Could you check a few things on this drawing? It's one solid part, dimensions in mm from its lowest x, y, z. A direction names the side the tool comes from. Give positions to 0.01 mm unless a question says otherwise; leave off trailing zeros. Write each loop counter-clockwise with the first axis right and the second up, starting at its lowest first coordinate (ties: lowest second). Pieces come first, ordered by that corner, then holes. Notation, with made-up numbers: M -2,-26.5 L 49,-26.5 A32 ccw 49,9.5 Z; hole C 62.25,72.25 d8. An arc over 180 degrees is marked long. Answer as CSV lines item,"result". Start each with the question number.
Q1. Suppose I cut it at C-C (y = 19.25). Write out the boundary of the cut face in (x, z).
Q2. Thinking about a two-plate mould opening in Z: for the marked faces 3, 4 and 5, which applies, +Z half, -Z half, draft (parallel to the pull), parting line (faces both ways), or undercut?
Q3. On a 3-axis mill with a long thin cutter (end or side, diameter ignored), from which of +Z, -Z, +X, -X, +Y, -Y can I reach the whole of each face in a straight line? I mean the marked faces 1 and 2. Say none if no direction works.
Q4. Suppose I cut it at A-A (z = 28). Write out the boundary of the cut face in (x, y), then the cut area to 3 significant figures.
Q5. If I drill on line 1 along Z through (x, y) = (11, 23); line 2 along X through (y, z) = (26.75, 13.5); line 3 along Y through (x, z) = (43.5, 18.5), over which ranges is the centre line in solid material (lowest first)?
Q6. Suppose I cut it at B-B (x = 29.5). Write out the boundary of the cut face in (y, z).
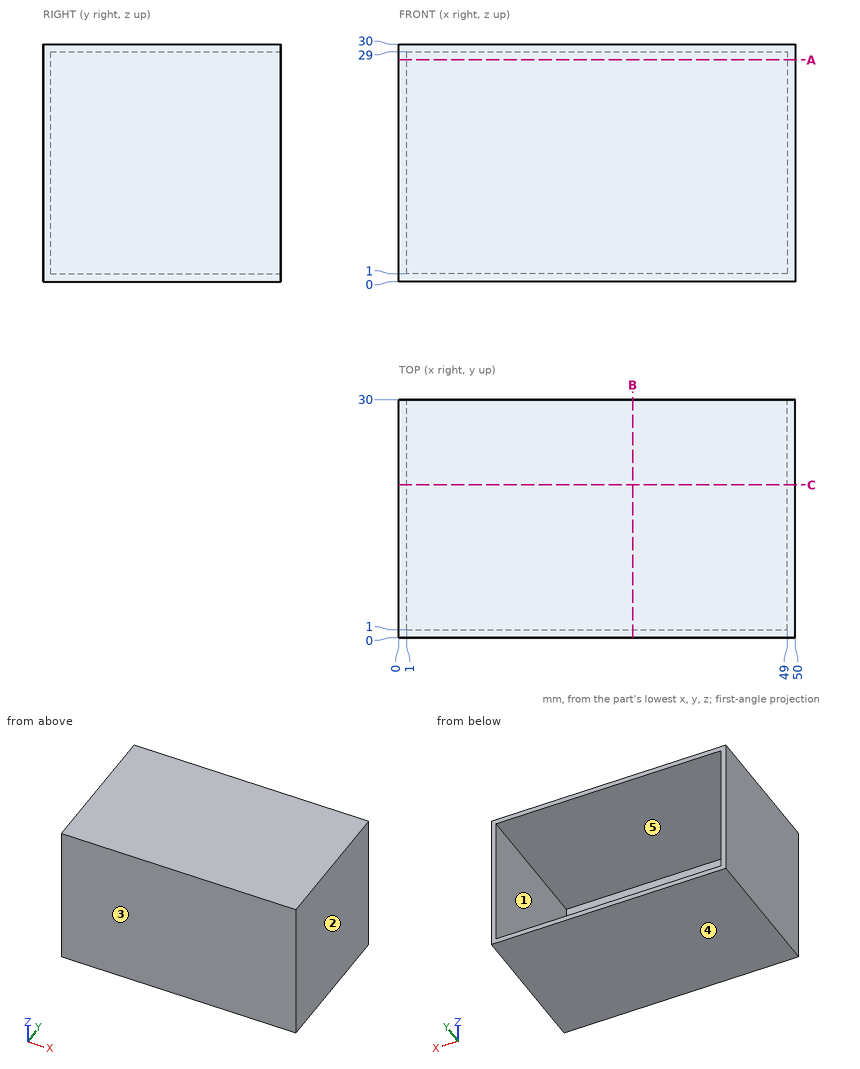
Resolved:
1,outline,"M 0,0 L 50,0 L 50,30 L 0,30 Z; hole M 1,1 L 49,1 L 49,29 L 1,29 Z"
2,face 3,"draft"
2,face 4,"-Z half"
2,face 5,"undercut"
3,face 1,"+Y"
3,face 2,"+Z, -Z, +X, +Y, -Y"
4,outline,"M 0,0 L 50,0 L 50,30 L 49,30 L 49,1 L 1,1 L 1,30 L 0,30 Z"
4,area,"108 mm^2"
5,line 1,"0 to 1, 29 to 30"
5,line 2,"0 to 1, 49 to 50"
5,line 3,"0 to 1"
6,outline,"M 0,0 L 30,0 L 30,1 L 1,1 L 1,29 L 30,29 L 30,30 L 0,30 Z"
